Geometry check sheet. Reference: the model listing, model coordinates, mm. A direction names the side the tool comes from. Give positions to 0.01 mm unless a question says otherwise; leave off trailing zeros. Loops run counter-clockwise (first coordinate to the right, second up) from the corner with the lowest first, then second, coordinate; pieces in that order, holes last.
1. Material ranges on L1, parallel to Y at x = 2.9, z = 2.5; L2, parallel to Z at x = 1.4, y = 0.25; L3, parallel to Z at x = 0.5, y = 0.75, recorded low to high.
2. Go/stop test with flat-tipped pins: pin 1 Ø1.8 at (y, z) = (0, 0) entering from +X; pin 2 Ø1 at (x, z) = (2.5, -1.5) entering from +Y. Record where each tip stops, or that it passes through.
3. Tool access check on faces 4 (the cylindrical face through (2.465, 2.524, 1.208)), 5 (the cylindrical face through (2.465, -2.524, -1.208)), 6 (the cylindrical face through (2.46, -1.94, -2.03)). Record the directions out of +Z, -Z, +X, -X, +Y, -Y that give a thin tool (end or side, any length) a straight path to the whole face; none if there is none.
4. Release check for a two-part mould opening along Z. For faces 1 (the flat face through (5, -1.2, 0)), 2 (the cylindrical face through (2.465, 1.929, -2.027)), 3 (the cylindrical face through (2.465, 2.752, -0.506)) record: +Z half, -Z half, draft (parallel to the pull), parting line (faces both ways), or undercut.
5. Cross-section at A-A, the plane z = 0. Record the cut outline in (x, y), plus the area to 3 significant figures.
from build123d import *

# Parameters (mm, degrees)
SKETCH2_R           = 2.2
SKETCH2_R_2         = 1
BOSS_EXTRUDE2_DEPTH = 5
BOSS_EXTRUDE3_DEPTH = 5
CIRPATTERN1_COUNT   = 10


with BuildPart() as part:
    # Sketch2 → Boss-Extrude2 (new body)
    with BuildSketch(Plane(origin=(0, 0, 0), x_dir=(0, 0, -1), z_dir=(1, 0, 0))):
        Circle(SKETCH2_R)
        Circle(SKETCH2_R_2, mode=Mode.SUBTRACT)
    extrude(amount=BOSS_EXTRUDE2_DEPTH)


with BuildPart() as body_2:
    # Sketch3 → Boss-Extrude3 (new body)
    with BuildSketch(Plane(origin=(0, 0, 0), x_dir=(0, 0, -1), z_dir=(1, 0, 0))):
        with BuildLine():
            ThreePointArc((-0.627770898, 2.108531171), (0, 2.2), (0.627770898, 2.108531171))
            Line((0.627770898, 2.108531171), (0.627770898, 2.212668909))
            ThreePointArc((0.627770898, 2.212668909), (0.502708566, 2.758930187), (0.15243605, 3.196367196))
            ThreePointArc((0.15243605, 3.196367196), (0, 3.2), (-0.15243605, 3.196367196))
            ThreePointArc((-0.15243605, 3.196367196), (-0.502708566, 2.758930187), (-0.627770898, 2.212668909))
            Line((-0.627770898, 2.212668909), (-0.627770898, 2.108531171))
        make_face()
    extrude(amount=BOSS_EXTRUDE3_DEPTH)


with BuildPart() as cirpattern1_1:
    # CirPattern1: pattern copy
    add(body_2.part.rotate(Axis((0, 0, 0), (1, 0, 0)), 1 * 360 / CIRPATTERN1_COUNT))


with BuildPart() as cirpattern1_2:
    # CirPattern1: pattern copy
    add(body_2.part.rotate(Axis((0, 0, 0), (1, 0, 0)), 2 * 360 / CIRPATTERN1_COUNT))


with BuildPart() as cirpattern1_3:
    # CirPattern1: pattern copy
    add(body_2.part.rotate(Axis((0, 0, 0), (1, 0, 0)), 3 * 360 / CIRPATTERN1_COUNT))


with BuildPart() as cirpattern1_4:
    # CirPattern1: pattern copy
    add(body_2.part.rotate(Axis((0, 0, 0), (1, 0, 0)), 4 * 360 / CIRPATTERN1_COUNT))


with BuildPart() as cirpattern1_5:
    # CirPattern1: pattern copy
    add(body_2.part.rotate(Axis((0, 0, 0), (1, 0, 0)), 5 * 360 / CIRPATTERN1_COUNT))


with BuildPart() as cirpattern1_6:
    # CirPattern1: pattern copy
    add(body_2.part.rotate(Axis((0, 0, 0), (1, 0, 0)), 6 * 360 / CIRPATTERN1_COUNT))


with BuildPart() as cirpattern1_7:
    # CirPattern1: pattern copy
    add(body_2.part.rotate(Axis((0, 0, 0), (1, 0, 0)), 7 * 360 / CIRPATTERN1_COUNT))


with BuildPart() as cirpattern1_8:
    # CirPattern1: pattern copy
    add(body_2.part.rotate(Axis((0, 0, 0), (1, 0, 0)), 8 * 360 / CIRPATTERN1_COUNT))


with BuildPart() as cirpattern1_9:
    # CirPattern1: pattern copy
    add(body_2.part.rotate(Axis((0, 0, 0), (1, 0, 0)), 9 * 360 / CIRPATTERN1_COUNT))


with BuildPart() as body_2_1:
    add(body_2.part)

    # Combine1: union CirPattern1_7, CirPattern1_6, CirPattern1_4, CirPattern1_3, part, CirPattern1_1, CirPattern1_2, CirPattern1_5, CirPattern1_8, CirPattern1_9
    add(cirpattern1_7.part)
    add(cirpattern1_6.part)
    add(cirpattern1_4.part)
    add(cirpattern1_3.part)
    add(part.part)
    add(cirpattern1_1.part)
    add(cirpattern1_2.part)
    add(cirpattern1_5.part)
    add(cirpattern1_8.part)
    add(cirpattern1_9.part)

    # Sketch4 → Cut-Revolve1 (revolve, cut)
    with BuildSketch(Plane.XY):
        Polygon((0, 0), (0, 2.8), (0.4, 3.2), (4.6, 3.2), (5, 2.8), (5, 0), (6, 0), (6, 4.2), (-1, 4.2), (-1, 0), align=None)
    revolve(axis=Axis((6, 0, 0), (-1, 0, 0)), mode=Mode.SUBTRACT)


solid = body_2_1.part
Result:
1. L1: y = -1.33 to -0.17, 0.17 to 1.33
1. L2: z = -2.63 to -0.97, 0.97 to 2.63
1. L3: z = -3.05 to -0.66, 0.66 to 3.05
2. pin 1: passes through
2. pin 2: stops at y = 2.68
3. face 4: +X, -X, +Y
3. face 5: +X, -X, -Y
3. face 6: -Z, +X, -X
4. face 1: draft
4. face 2: -Z half
4. face 3: undercut
5. outline: (0, -2.8) - (0.4, -3.2) - (4.6, -3.2) - (5, -2.8) - (5, -1) - (0, -1) - close; (0, 1) - (5, 1) - (5, 2.8) - (4.6, 3.2) - (0.4, 3.2) - (0, 2.8) - close
5. area: 21.7 mm2
